from build123d import *

# Parameters (mm, degrees)
SKETCH1_W           = 150
SKETCH1_H           = 150
BOSS_EXTRUDE1_DEPTH = 60
SHELL1_T            = -7.5
SKETCH5_R           = 2.5
CUT_EXTRUDE2_DEPTH  = 10
SKETCH6_R           = 1.5
CUT_EXTRUDE3_DEPTH  = 10


with BuildPart() as part:
    # Sketch1 → Boss-Extrude1 (new body)
    with BuildSketch(Plane(origin=(0, 0, 0), x_dir=(1, 0, 0), z_dir=(0, 1, 0))):
        Rectangle(SKETCH1_W, SKETCH1_H)
    extrude(amount=BOSS_EXTRUDE1_DEPTH)

    # Shell1
    shell1_openings = [part.faces().sort_by_distance(p)[0] for p in [
        (0, 0, 0),
    ]]
    offset(amount=SHELL1_T, openings=shell1_openings, kind=Kind.INTERSECTION)

    # Sketch5 → Cut-Extrude2 (cut)
    with BuildSketch(Plane.XY.offset(75)):
        with Locations((-50, 5)):
            Circle(SKETCH5_R)
        with Locations((-40, 5)):
            Circle(SKETCH5_R)
        with Locations((-30, 5)):
            Circle(SKETCH5_R)
        with Locations((30, 5)):
            Circle(SKETCH5_R)
        with Locations((40, 5)):
            Circle(SKETCH5_R)
        with Locations((50, 5)):
            Circle(SKETCH5_R)
    extrude(amount=-CUT_EXTRUDE2_DEPTH, mode=Mode.SUBTRACT)

    # Sketch6 → Cut-Extrude3 (cut)
    with BuildSketch(Plane(origin=(0, 0, -75), x_dir=(-1, 0, 0), z_dir=(0, 0, -1))):
        with Locations((-14.5, 8)):
            Circle(SKETCH6_R)
        with Locations((14.5, 8)):
            Circle(SKETCH6_R)
    extrude(amount=-CUT_EXTRUDE3_DEPTH, mode=Mode.SUBTRACT)


solid = part.part
Work out the finished part from the listing and answer in its coordinate system (mm). A direction names the side the tool comes from. Coordinates: 2 decimals unless noted, no trailing zeros. Loops run counter-clockwise (first coordinate to the right, second up) from the corner with the lowest first, then second, coordinate; pieces in that order, holes last. Notation, with made-up numbers: M 10,0 L 54,0 A11 ccw 54,10 Z; hole C 75.5,-29.5 d10. An arc over 180 degrees is marked long. Answer in a Markdown table with one row per item. Add a question column.
1. Find section A-A, the plane y = 12. Write down the section's boundary in (x, z), then the cut area to 4 significant figures.
2. The mould has two halves that part along Y. Classify faces 4 (the flat face through (-1, 52.5, -1)), 5 (the cylindrical face through (-37.69, 4.04, 71.3)), 6 (the flat face through (-1, 60, -1)): pulls with the +Y half, pulls with the -Y half, needs draft (parallel to the pull), parting line crosses it, or undercut.
3. Consider L1, parallel to Z at x = -25.5, y = 31; L2, parallel to Y at x = 40, z = 71.5. Determine where each line is inside the solid, lowest interval first.
4. Find section B-B, the plane x = 30. Write down the section's boundary in (y, z), then the cut area to 4 significant figures.
5. Flat-ended cylindrical pins translate along their axes: P1, Ø3, axis at x = 40, y = 5, coming from the +Z side; P2, Ø2, axis at x = 2.5, z = 55.5, coming from the -Y side. Find the tip coordinate at first contact, or state that the pin passes through.
6. Find section C-C, the plane z = -34. Write down the section's boundary in (x, y), then the cut area to 3 significant figures.
7. A tool of negligible diameter and unlimited length cuts with its end or side. For faces 1 (the flat face through (-1, 30, -75)), 2 (the cylindrical face through (52.31, 4.04, 71.3)), 3 (the flat face through (67.5, 26, 1)), from which of +Z, -Z, +X, -X, +Y, -Y can it reach the whole face along a straight path? Write none if from no direction.
Reported:
| question | item | result |
|---|---|---|
| 1 | outline | M -75,-75 L 75,-75 L 75,75 L -75,75 Z; hole M -67.5,-67.5 L 67.5,-67.5 L 67.5,67.5 L -67.5,67.5 Z |
| 1 | area | 4,275 mm^2 |
| 2 | face 4 | pulls with the -Y half |
| 2 | face 5 | undercut |
| 2 | face 6 | pulls with the +Y half |
| 3 | L1 | z = -75 to -67.5, 67.5 to 75 |
| 3 | L2 | y = 0 to 2.5, 7.5 to 60 |
| 4 | outline | M 0,-75 L 60,-75 L 60,75 L 7.5,75 L 7.5,67.5 L 52.5,67.5 L 52.5,-67.5 L 0,-67.5 Z; M 0,67.5 L 2.5,67.5 L 2.5,75 L 0,75 Z |
| 4 | area | 1,875 mm^2 |
| 5 | P1 | stops at z = -67.5 |
| 5 | P2 | stops at y = 52.5 |
| 6 | outline | M -75,0 L -67.5,0 L -67.5,52.5 L 67.5,52.5 L 67.5,0 L 75,0 L 75,60 L -75,60 Z |
| 6 | area | 1,910 mm^2 |
| 7 | face 1 | -Z, +X, -X, +Y, -Y |
| 7 | face 2 | +Z |
| 7 | face 3 | -Y |
